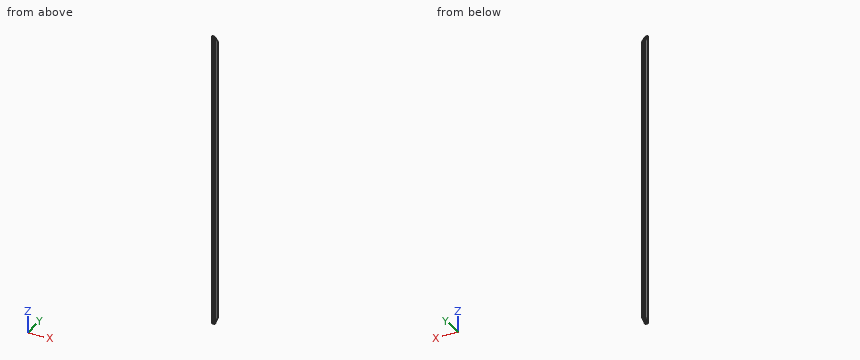
Autodesk Inventor part; units mm, degrees
ref_plane "Start plane" through (0, 0, 0) normal (0, 0, 1) x (1, 0, 0)
ref_plane "End plane" through (0, 0, 2000) normal (0, 0, 1) x (1, 0, 0)
ref_plane "YZ Plane" through (0, 0, 0) normal (1, 0, 0) x (0, 1, 0)
ref_plane "Start plane" through (0, 0, 0) normal (0, 0, 1) x (1, 0, 0)
ref_plane "End plane" through (0, 0, 2000) normal (0, 0, 1) x (1, 0, 0)
sketch "Sketch" plane through (0, 0, 0) normal (0, 0, 1) x (1, 0, 0)
  line L0 (-10, -16) -> (-10, 16)
  line L1 (-6, 20) -> (6, 20)
  line L2 (10, 16) -> (10, -16)
  line L3 (6, -20) -> (-6, -20)
  arc A0 (-10, -16) -> (-6, -20) centre (-6, -16) ccw
  arc A1 (10, 16) -> (6, 20) centre (6, 16) ccw
  arc A2 (-6, 20) -> (-10, 16) centre (-6, 16) ccw
  arc A3 (6, -20) -> (10, -16) centre (6, -16) ccw
  arc A4 (-6, 18) -> (-8, 16) centre (-6, 16) ccw
  line L4 (-6, 18) -> (6, 18)
  arc A5 (8, 16) -> (6, 18) centre (6, 16) ccw
  line L5 (8, 16) -> (8, -16)
  arc A6 (6, -18) -> (8, -16) centre (6, -16) ccw
  line L6 (6, -18) -> (-6, -18)
  arc A7 (-8, -16) -> (-6, -18) centre (-6, -16) ccw
  line L7 (-8, -16) -> (-8, 16)
  line L8 (0, 29.1598) -> (0, -29.1598) construction
  line L9 (-15.1598, 0) -> (15.1598, 0) construction
  dimension "d7" = 4
  dimension "d9" = 20
  dimension "d11" = 40
  dimension "d12" = 2
  dimension "d15" = 10
  dimension "d16" = 20
extrude "Body" add sketch "Sketch" along normal up to surface (2000 mm away) from surface at 0
sketch "Sketch3" plane through (0, 0, 0) normal (0, 0, 1) x (1, 0, 0)
  line L0 (0, 0) -> (10, 0)
ref_plane "Work Plane3" through (0, 0, 0) normal (0, -1, 0) x (1, 0, 0)
sketch "Sketch5" plane through (0, 0, 0) normal (1, 0, 0) x (0, 1, 0)
  line L0 (-20, 0) -> (-20, 2000)
  line L1 (-20, 0) -> (-20, 2000)
  line L2 (20, 0) -> (20, 2000)
  line L3 (20, 0) -> (20, 2000)
  line L4 (-20, 0) -> (20, 0)
  line L5 (20, 2000) -> (-20, 2000)
  line L6 (-20, 2000) -> (20, 1942.8741)
  line L7 (-20, 0) -> (20, 28.0083)
  point P0 (0, 0)
  point P1 (20, 28.0083)
  point P2 (20, 1942.8741)
  dimension "d19" = 55
  dimension "d20" = 35
extrude "Extrusion2" cut sketch "Sketch5" along normal through all both and the other way through all contours L7 L2 L4 | L5 L2 L6
sketch "Sketch4" plane through (0, 0, 0) normal (0, -1, 0) x (1, 0, 0)
  line L0 (-2, 0) -> (12, 0)
  line L1 (-2, 2000) -> (12, 2000)
  dimension "d18" = 2000
equation "\"d7\" = G_IR"
equation "\"d9\" = G_W"
equation "\"d11\" = G_H"
equation "\"d12\" = G_T"
equation "\"d15\" = 0.5 * d9"
equation "\"d16\" = 0.5 * d11"
equation "\"d3\" = G_L"
equation "\"G_W\" = 20"
equation "\"G_H\" = 40"
equation "\"G_T\" = 2"
equation "\"G_IR\" = 4"
equation "\"G_L\" = d18"
equation "\"G_OFFSET_START\" = 0"
equation "\"G_OFFSET_END\" = 0"
properties part number "ISO 4019 - 40x20x2 - 2000" material "Steel, Mild"
Design review of the part built by this model. Coordinates are the model's own, in mm. Round coordinates to 2 decimals unless told otherwise and drop trailing zeros. Order: outer loops, then holes, each group sorted by start corner. A loop starts at its lowest first (then second) coordinate and runs counter-clockwise, first axis right, second up.
1) Consider section A-A (x = 0). State the section outline as (y, z) points.
The answers:
outline: (-20, 0) - (-18, 1.4) - (-18, 1997.14) - (-20, 2000) - close; (18, 26.61) - (20, 28.01) - (20, 1942.87) - (18, 1945.73) - close
2) For L1, parallel to X at y = -8, z = 234.5; L2, parallel to Y at x = 1.75, z = 1524.5; L3, parallel to Y at x = 6.75, z = 711.5, list the stretches that pass through material, from the lowest coordinate up.
The answers:
L1: x = -10 to -8, 8 to 10
L2: y = -20 to -18, 18 to 20
L3: y = -19.93 to -17.85, 17.85 to 19.93
3) Consider section B-B (y = -8). State the section outline as (x, z) points.
The answers:
outline: (-10, 8.4) - (-8, 8.4) - (-8, 1982.86) - (-10, 1982.86) - close; (8, 8.4) - (10, 8.4) - (10, 1982.86) - (8, 1982.86) - close
4) Clearance check with flat-ended pins moving along their axes: pin 1 Ø1 at (x, y) = (8, -5.5) entering from +Z; pin 2 Ø8 at (x, y) = (-1, 4.5) entering from +Z. State where each tip first meets the part, or that it passes through.
The answers:
pin 1: stops at z = 1980.01
pin 2: passes through
5) Consider section C-C (z = 1691). State the section outline as (x, y) points, plus the area to 3 significant figures.
The answers:
outline: (-10, -16) arc R4 ccw to (-6, -20) - (6, -20) arc R4 ccw to (10, -16) - (10, 16) arc R4 ccw to (6, 20) - (-6, 20) arc R4 ccw to (-10, 16) - close; hole (-8, -16) arc R2 ccw to (-6, -18) - (6, -18) arc R2 ccw to (8, -16) - (8, 16) arc R2 ccw to (6, 18) - (-6, 18) arc R2 ccw to (-8, 16) - close
area: 214 mm2
